from build123d import *

# Parameters (mm, degrees)
SKETCH_W        = 220
SKETCH_H        = 40
PAD_DEPTH       = 10
SKETCH001_R     = 19
POCKET_DEPTH    = 10
PAD001_DEPTH    = 220
PAD002_DEPTH    = 220
SKETCH004_R     = 1.325
POCKET001_DEPTH = 10
SKETCH005_R     = 1.325
POCKET002_DEPTH = 10
SKETCH006_W     = 106.6
SKETCH006_H     = 10
PAD003_DEPTH    = 70
SKETCH007_W     = 19.8
SKETCH007_H     = 10
POCKET003_DEPTH = 30
SKETCH008_W     = 56.7
SKETCH008_H     = 10
PAD004_DEPTH    = 8
SKETCH009_W     = 56.7
SKETCH009_H     = 8
PAD005_DEPTH    = 20
SKETCH010_R     = 2.375
POCKET004_DEPTH = 10
POCKET005_DEPTH = 4
FILLET_R        = 5
SKETCH012_R     = 1.75
POCKET006_DEPTH = 8
SKETCH013_R     = 2.875
POCKET007_DEPTH = 4
SKETCH014_R     = 1.325
POCKET008_DEPTH = 10
SKETCH015_W     = 72
SKETCH015_H     = 7
POCKET009_DEPTH = 10
FILLET001_R     = 2
SKETCH016_W     = 220
SKETCH016_H     = 10
PAD006_DEPTH    = 3
CHAMFER_SIZE    = 2.99


with BuildPart() as part:
    # Sketch → Pad (new body)
    with BuildSketch(Plane.XY):
        Rectangle(SKETCH_W, SKETCH_H)
    extrude(amount=PAD_DEPTH)

    # Sketch001 (on Face6 of Pad) → Pocket (cut)
    with BuildSketch(Plane.XY.offset(10)):
        with Locations((-80, 0)):
            Circle(SKETCH001_R)
        with Locations((-40, 0)):
            Circle(SKETCH001_R)
        Circle(SKETCH001_R)
        with Locations((40, 0)):
            Circle(SKETCH001_R)
        with Locations((80, 0)):
            Circle(SKETCH001_R)
    extrude(amount=-POCKET_DEPTH, mode=Mode.SUBTRACT)

    # Sketch002 (on Face3 of Pocket) → Pad001 (join)
    with BuildSketch(Plane.YZ.offset(110)):
        Polygon((-10, 0), (-20, 0), (-20, 10), align=None)
    extrude(amount=-PAD001_DEPTH)

    # Sketch003 (on Face3 of Pad001) → Pad002 (join)
    with BuildSketch(Plane.YZ.offset(110)):
        Polygon((20, 10), (10, 0), (20, 0), align=None)
    extrude(amount=-PAD002_DEPTH)

    # Sketch004 (on Face5 of Pad002) → Pocket001 (cut)
    with BuildSketch(Plane.XY.offset(10)):
        with Locations((-96, 16)):
            Circle(SKETCH004_R)
        with Locations((-96, -16)):
            Circle(SKETCH004_R)
        with Locations((-64, -16)):
            Circle(SKETCH004_R)
        with Locations((-64, 16)):
            Circle(SKETCH004_R)
        with Locations((-56, 16)):
            Circle(SKETCH004_R)
        with Locations((-56, -16)):
            Circle(SKETCH004_R)
        with Locations((-24, -16)):
            Circle(SKETCH004_R)
        with Locations((-24, 16)):
            Circle(SKETCH004_R)
        with Locations((-16, 16)):
            Circle(SKETCH004_R)
        with Locations((-16, -16)):
            Circle(SKETCH004_R)
        with Locations((16, -16)):
            Circle(SKETCH004_R)
        with Locations((16, 16)):
            Circle(SKETCH004_R)
        with Locations((24, 16)):
            Circle(SKETCH004_R)
        with Locations((24, -16)):
            Circle(SKETCH004_R)
        with Locations((56, -16)):
            Circle(SKETCH004_R)
        with Locations((56, 16)):
            Circle(SKETCH004_R)
        with Locations((64, 16)):
            Circle(SKETCH004_R)
        with Locations((64, -16)):
            Circle(SKETCH004_R)
        with Locations((96, -16)):
            Circle(SKETCH004_R)
        with Locations((96, 16)):
            Circle(SKETCH004_R)
    extrude(amount=-POCKET001_DEPTH, mode=Mode.SUBTRACT)

    # Sketch005 (on Face5 of Pocket001) → Pocket002 (cut)
    with BuildSketch(Plane.XY.offset(10)):
        with Locations((-105, 10)):
            Circle(SKETCH005_R)
        with Locations((-105, -10)):
            Circle(SKETCH005_R)
        with Locations((105, 10)):
            Circle(SKETCH005_R)
        with Locations((105, -10)):
            Circle(SKETCH005_R)
    extrude(amount=-POCKET002_DEPTH, mode=Mode.SUBTRACT)

    # Sketch006 (on Face1 of Pocket002) → Pad003 (join)
    with BuildSketch(Plane(origin=(0, 20, 0), x_dir=(-1, 0, 0), z_dir=(0, 1, 0))):
        with Locations((0, 5)):
            Rectangle(SKETCH006_W, SKETCH006_H)
    extrude(amount=PAD003_DEPTH)

    # Sketch007 → Pocket003 (cut)
    with BuildSketch(Plane(origin=(0, 90, 0), x_dir=(-1, 0, 0), z_dir=(0, 1, 0))):
        with Locations((-43.4, 5)):
            Rectangle(SKETCH007_W, SKETCH007_H)
        with Locations((43.4, 5)):
            Rectangle(SKETCH007_W, SKETCH007_H)
    extrude(amount=-POCKET003_DEPTH, mode=Mode.SUBTRACT)

    # Sketch008 (on Face1 of Pocket003) → Pad004 (join)
    with BuildSketch(Plane(origin=(0, 20, 0), x_dir=(-1, 0, 0), z_dir=(0, 1, 0))):
        with Locations((-81.65, 5)):
            Rectangle(SKETCH008_W, SKETCH008_H)
        with Locations((81.65, 5)):
            Rectangle(SKETCH008_W, SKETCH008_H)
    extrude(amount=PAD004_DEPTH)

    # Sketch009 (on Face14 of Pad004) → Pad005 (join)
    with BuildSketch(Plane(origin=(0, 0, 0), x_dir=(1, 0, 0), z_dir=(0, 0, -1))):
        with Locations((-81.65, -24)):
            Rectangle(SKETCH009_W, SKETCH009_H)
        with Locations((81.65, -24)):
            Rectangle(SKETCH009_W, SKETCH009_H)
    extrude(amount=PAD005_DEPTH)

    # Sketch010 (on Face15 of Pad005) → Pocket004 (cut)
    with BuildSketch(Plane(origin=(0, 0, 0), x_dir=(1, 0, 0), z_dir=(0, 0, -1))):
        with Locations((-28, -75)):
            Circle(SKETCH010_R)
        with Locations((28, -75)):
            Circle(SKETCH010_R)
    extrude(amount=-POCKET004_DEPTH, mode=Mode.SUBTRACT)

    # Sketch011 (on Face87 of Pocket004) → Pocket005 (cut)
    with BuildSketch(Plane.XY.offset(10)):
        Polygon((-24.35, 72.892672), (-24.35, 77.107328), (-28, 79.214657), (-31.65, 77.107328), (-31.65, 72.892672), (-28, 70.785343), align=None)
        Polygon((31.65, 77.107328), (28, 79.214657), (24.35, 77.107328), (24.35, 72.892672), (28, 70.785343), (31.65, 72.892672), align=None)
    extrude(amount=-POCKET005_DEPTH, mode=Mode.SUBTRACT)

    # Fillet
    fillet_edges = [part.edges().sort_by_distance(p)[0] for p in [
        (53.3, 60, 5),
        (-53.3, 60, 5),
    ]]
    fillet(fillet_edges, radius=FILLET_R)

    # Sketch012 (on Face19 of Fillet) → Pocket006 (cut)
    with BuildSketch(Plane(origin=(0, 28, 0), x_dir=(-1, 0, 0), z_dir=(0, 1, 0))):
        with Locations((-100, -10)):
            Circle(SKETCH012_R)
        with Locations((-65, -10)):
            Circle(SKETCH012_R)
        with Locations((65, -10)):
            Circle(SKETCH012_R)
        with Locations((100, -10)):
            Circle(SKETCH012_R)
    extrude(amount=-POCKET006_DEPTH, mode=Mode.SUBTRACT)

    # Sketch013 (on Face19 of Pocket006) → Pocket007 (cut)
    with BuildSketch(Plane(origin=(0, 28, 0), x_dir=(-1, 0, 0), z_dir=(0, 1, 0))):
        with Locations((-100, -10)):
            Circle(SKETCH013_R)
        with Locations((-65, -10)):
            Circle(SKETCH013_R)
        with Locations((65, -10)):
            Circle(SKETCH013_R)
        with Locations((100, -10)):
            Circle(SKETCH013_R)
    extrude(amount=-POCKET007_DEPTH, mode=Mode.SUBTRACT)

    # Sketch014 (on Face17 of Pocket007) → Pocket008 (cut)
    with BuildSketch(Plane.XY.offset(10)):
        with Locations((-10, 85)):
            Circle(SKETCH014_R)
        with Locations((10, 85)):
            Circle(SKETCH014_R)
    extrude(amount=-POCKET008_DEPTH, mode=Mode.SUBTRACT)

    # Sketch015 (on Face19 of Pocket008) → Pocket009 (cut)
    with BuildSketch(Plane.XY.offset(10)):
        with Locations((0, 35.5)):
            Rectangle(SKETCH015_W, SKETCH015_H)
    extrude(amount=-POCKET009_DEPTH, mode=Mode.SUBTRACT)

    # Fillet001
    fillet001_edges = [part.edges().sort_by_distance(p)[0] for p in [
        (36, 39, 5),
        (-36, 39, 5),
        (-36, 32, 5),
        (36, 32, 5),
    ]]
    fillet(fillet001_edges, radius=FILLET001_R)

    # Sketch016 (on Face104 of Fillet001) → Pad006 (join)
    with BuildSketch(Plane.XZ.offset(20)):
        with Locations((0, 5)):
            Rectangle(SKETCH016_W, SKETCH016_H)
    extrude(amount=PAD006_DEPTH)

    # Chamfer
    chamfer_edges = [part.edges().sort_by_distance(p)[0] for p in [
        (0, -23, 0),
    ]]
    chamfer(chamfer_edges, length=CHAMFER_SIZE)


solid = part.part
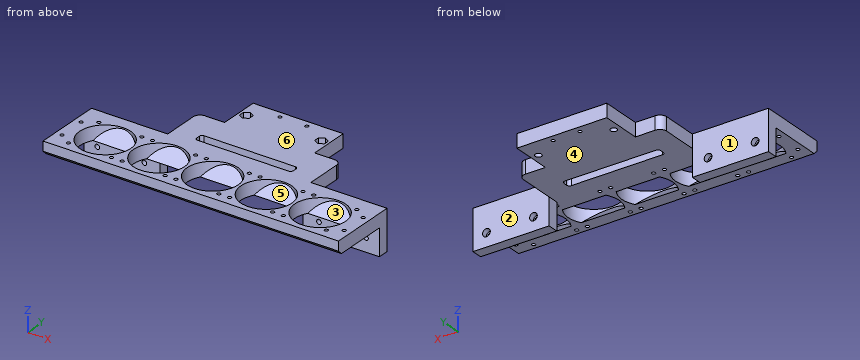
Read the model definition and answer for the solid it produces. Units are mm, in the model's axes. Face numbers are marked on the shaded views. A direction names the side the tool comes from. Give positions to 0.01 mm unless a question says otherwise; leave off trailing zeros. Write each loop counter-clockwise with the first axis right and the second up, starting at its lowest first coordinate (ties: lowest second). Pieces come first, ordered by that corner, then holes. Notation, with made-up numbers: (-4, 21.25) - (18, 21.25) arc R15 ccw to (18, 25.25) - close; hole circle Ø10 at (62, 38.5). An arc over 180 degrees is marked (long way). Use CSV: the item, a comma, the result in double quotes. Start each with the question number.
(1) Given P1, Ø8, axis at x = -41.5, z = 7, coming from the +Y side; P2, Ø1.7, axis at x = 99, z = -11, coming from the +Y side; P3, Ø4, axis at y = 74.5, z = 2.5, coming from the +X side, each flat-ended and moving along its own axis, determine where each tip first touches the part or whether it passes through.
(2) Find section A-A (y = 0). Give the vertices of the cut face in (x, z), plus the area to 3 significant figures.
(3) Find section B-B (z = -3.5). Give the vertices of the cut face in (x, y), plus the area to 3 significant figures.
(4) For the marked faces 1, 2, 3 and 4, determine the directions among +Z, -Z, +X, -X, +Y, -Y from which every point of the face is accessible in a straight line to the end or side of a thin tool.
(5) Consider line 1 along X through (y, z) = (0, 7.5); line 2 along X through (y, z) = (26, -7.75); line 3 along Y through (x, z) = (-28, 1.9) (3 decimals). Determine where each line is inside the solid, lowest interval first.
(6) Determine the mould class of the marked faces 5 and 6 for opening direction X: +X half, -X half, draft (parallel to the pull), parting line (faces both ways), or undercut.
(7) Find section D-D (y = 58). Give the vertices of the cut face in (x, z), plus the area to 3 significant figures.
(8) Find section C-C (x = -90.5). Give the vertices of the cut face in (y, z).
Findings below:
1,P1,"y = 60"
1,P2,"y = 24"
1,P3,"x = 33.5"
2,outline,"(-110, 0) - (-99, 0) - (-99, 10) - (-110, 10) - close; (-61, 0) - (-59, 0) - (-59, 10) - (-61, 10) - close; (-21, 0) - (-19, 0) - (-19, 10) - (-21, 10) - close; (19, 0) - (21, 0) - (21, 10) - (19, 10) - close; (59, 0) - (61, 0) - (61, 10) - (59, 10) - close; (99, 0) - (110, 0) - (110, 10) - (99, 10) - close"
2,area,"300 mm2"
3,outline,"(-110, 20) - (-53.3, 20) - (-53.3, 28) - (-110, 28) - close; (53.3, 20) - (110, 20) - (110, 28) - (53.3, 28) - close"
3,area,"907 mm2"
4,face 1,"+Z, -Z, -X, +Y"
4,face 2,"+Z, -Z, +X, +Y"
4,face 3,"+Z"
4,face 4,"-Z, -Y"
5,line 1,"-110 to -99, -61 to -59, -21 to -19, 19 to 21, 59 to 61, 99 to 110"
5,line 2,"-110 to -101.79, -98.21 to -66.79, -63.21 to -53.3, 53.3 to 63.21, 66.79 to 98.21, 101.79 to 110"
5,line 3,"-21.91 to -11.9, 11.9 to 32, 39 to 72.625, 77.375 to 90"
6,face 5,"undercut"
6,face 6,"draft"
7,outline,"(-52.3, 0) - (52.3, 0) - (52.3, 10) - (-52.3, 10) - close"
7,area,"1,050 mm2"
8,outline,"(-23, 2.99) - (-20.01, 0) - (-10, 0) - (-15.84, 5.84) - (-15.84, 10) - (-23, 10) - close; (10, 0) - (20, 0) - (20, -20) - (28, -20) - (28, 10) - (15.84, 10) - (15.84, 5.84) - close"
